from build123d import *

# Parameters (mm, degrees)
F1_W     = 9.5782261753
F1_H     = 9.891791337
F1_H_2   = 10.108208663
F1_W_2   = 10
F1_H_3   = 10
F2_DEPTH = 5
F3_W     = 10.1701691747
F3_H     = 1.1901259422
F3_W_2   = 2.3802500218
F3_W_3   = 1.1901250109
F3_H_2   = 0.8006438729
F3_H_3   = 10.4947462678
F3_W_4   = 5.1932781935
F3_H_4   = 1.9474774599
F3_W_5   = 1.1901259422
F3_H_5   = 8.5062488797
F3_W_6   = 9.7373928875
F3_W_7   = 1.514704898
F3_H_6   = 9.3068927526
F3_W_8   = 10.1330708712
F3_H_7   = 1.6025230289
F3_W_9   = 9.0882331133
F3_H_8   = 3.835350275
F3_W_10  = 1.0448377579
F3_H_9   = 8.595854044
F3_W_11  = 1.0108357528
F3_W_12  = 1.0278367554
F3_H_10  = 0.8937604725
F4_DEPTH = 25
F5_W     = 8.1058442593
F5_H     = 1.9299630076
F5_W_2   = 1.5439689159
F5_W_3   = 1.5439717099
F5_H_2   = 11.9657684118
F5_W_4   = 10.3005599231
F5_H_3   = 1.0513318703
F6_DEPTH = 25


# Not quite as in the source:
# - a feature names something its author has since deleted; it is built from what else it names


with BuildPart() as f2:
    # F1 (on Top) → F2 (new body)
    with BuildSketch(Plane.XY):
        with Locations((-4.7891130877, 4.9458956685)):
            Rectangle(F1_W, F1_H)
        Polygon((-10, 0), (-9.5782261753, 0), (-9.5782261753, 9.891791337), (-19.5782261753, 9.891791337), (-19.5782261753, 0), align=None)
        with Locations((-4.7891130877, 14.9458956685)):
            Rectangle(F1_W, F1_H_2)
        Polygon((0, 30), (0, 20), (0.4217738247, 20), (10, 20), (10, 30), align=None)
        Polygon((-9.5782261753, 20), (0, 20), (0, 30), (-10.0065707871, 30), align=None)
        with Locations((-24.5782261753, 4.9458956685)):
            Rectangle(F1_W_2, F1_H)
        with Locations((-24.5782261753, -5)):
            Rectangle(F1_W_2, F1_H_3)
        with BuildLine():
            Line((-10.0065707871, 30), (0, 30))
            Line((0, 30), (0, 44))
            ThreePointArc((0, 44), (-5.0363871882, 43.7108087787), (-10.0065707871, 42.8470365496))
            Line((-10.0065707871, 42.8470365496), (-10.0065707871, 30))
        make_face()
        with BuildLine():
            Line((-44, 0), (-29.5782261753, 0))
            Line((-29.5782261753, 0), (-29.5782261753, 9.891791337))
            add(Edge.make_bspline(
                [(-29.5782261753, 9.891791337), (-29.5956822452, 12.6865898133), (-29.4779762378, 16.6539770733), (-27.9306023487, 20)],
                knots=[0, 0, 0, 0, 0.3288616787, 0.3288616787, 0.3288616787, 0.3288616787], degree=3))
            Line((-27.9306023487, 20), (-39.1918358845, 20))
            ThreePointArc((-39.1918358845, 20), (-42.7810751321, 10.2849215136), (-44, 0))
        make_face()
        with BuildLine():
            add(Edge.make_bspline(
                [(-19.5782261753, 28.0459611928), (-16.4208018887, 29.540455447), (-13.1162348053, 30), (-10.0065707871, 30)],
                knots=[0.678814496, 0.678814496, 0.678814496, 0.678814496, 1, 1, 1, 1], degree=3))
            Line((-10.0065707871, 30), (-10.0065707871, 42.8470365496))
            ThreePointArc((-10.0065707871, 42.8470365496), (-14.8922224071, 41.4031606496), (-19.5782261753, 39.4042264209))
            Line((-19.5782261753, 39.4042264209), (-19.5782261753, 28.0459611928))
        make_face()
        with BuildLine():
            add(Edge.make_bspline(
                [(-24.5782261753, 24.6040217078), (-23.0917294817, 26.0318138691), (-21.358363516, 27.2033740757), (-19.5782261753, 28.0459611928)],
                knots=[0.497731988, 0.497731988, 0.497731988, 0.497731988, 0.678814496, 0.678814496, 0.678814496, 0.678814496], degree=3))
            Line((-19.5782261753, 28.0459611928), (-19.5782261753, 39.4042264209))
            ThreePointArc((-19.5782261753, 39.4042264209), (-23.9356591488, 36.9199704918), (-27.9820429197, 33.9559313529))
            Line((-27.9820429197, 33.9559313529), (-24.5782261753, 24.6040217078))
        make_face()
        with BuildLine():
            Line((-39.1918358845, 20), (-27.9306023487, 20))
            add(Edge.make_bspline(
                [(-27.9306023487, 20), (-27.136026622, 21.7181811177), (-25.9644735778, 23.2725198056), (-24.5782261753, 24.6040217078)],
                knots=[0.3288616787, 0.3288616787, 0.3288616787, 0.3288616787, 0.497731988, 0.497731988, 0.497731988, 0.497731988], degree=3))
            Line((-24.5782261753, 24.6040217078), (-33.9336129947, 28.00910404))
            ThreePointArc((-33.9336129947, 28.00910404), (-36.7813710365, 24.148100229), (-39.1918358845, 20))
        make_face()
        with BuildLine():
            Line((-33.9336129947, 28.00910404), (-24.5782261753, 24.6040217078))
            Line((-24.5782261753, 24.6040217078), (-27.9820429197, 33.9559313529))
            ThreePointArc((-27.9820429197, 33.9559313529), (-31.1002942205, 31.1250975806), (-33.9336129947, 28.00910404))
        make_face()
    extrude(amount=F2_DEPTH)

    # F3 (on offset) → F4 (cut)
    with BuildSketch(Plane.XY.offset(3)):
        Polygon((-33.0700390041, 9.3068927526), (-33.0700390041, 0), (-31.8799139932, 0), (-31.8799139932, 0.8006438729), (-30.6897889823, 0.8006438729), (-30.6897889823, 9.3068927526), align=None)
        with Locations((-38.1551235914, 9.9019557238)):
            Rectangle(F3_W, F3_H)
        with Locations((-31.8799139932, 9.9019557238)):
            Rectangle(F3_W_2, F3_H)
        with Locations((-31.2848514877, 0.4003219365)):
            Rectangle(F3_W_3, F3_H_2)
        Polygon((-30.6897889823, 0), (-31.8799139932, 0), (-31.8799139932, -0.8824482211), (-21.3851686567, -0.8824482211), (-21.3851686567, 0), (-22.5752945989, 0), (-22.5752945989, 0.8006438729), (-30.6897889823, 0.8006438729), align=None)
        with Locations((-31.8799139932, 15.7443918288)):
            Rectangle(F3_W_2, F3_H_3)
        with Locations((-35.6666781008, 21.9655036926)):
            Rectangle(F3_W_4, F3_H_4)
        Polygon((-33.0700390041, 22.9392424226), (-33.0700390041, 20.9917649627), (-30.6897889823, 20.9917649627), (-30.6897889823, 22.9392424226), (-31.3607603312, 22.9392424226), align=None)
        with Locations((-21.9802316278, 5.0537683128)):
            Rectangle(F3_W_5, F3_H_5)
        with Locations((-21.9802316278, 9.9019557238)):
            Rectangle(F3_W_5, F3_H)
        with Locations((-21.9802316278, 0.4003219365)):
            Rectangle(F3_W_5, F3_H_2)
        with Locations((-16.516472213, 9.9019557238)):
            Rectangle(F3_W_6, F3_H)
        Polygon((-29.9641676247, 26.1324569583), (-31.3607603312, 22.9392424226), (-30.6897889823, 22.9392424226), (-29.4176749885, 22.9392424226), (-28.3854100853, 25.160914287), (-27.413867414, 27.1647218615), (-25.7743895054, 28.682757169), (-24.2563541979, 29.8971850425), (-22.5752945989, 30.6865628809), (-22.5752945989, 31.9009907544), (-23.8920263946, 31.41522035), (-26.1387173086, 30.0793480128), (-26.8673747778, 29.40273819), (-26.8673747778, 27.7112144977), (-27.413867414, 27.7112144977), (-27.9603600502, 27.7112144977), (-28.6890175194, 27.7112144977), align=None)
        with Locations((-10.8904233202, 4.6534463763)):
            Rectangle(F3_W_7, F3_H_6)
        with Locations((-10.8904233202, 9.9019557238)):
            Rectangle(F3_W_7, F3_H)
        Polygon((-22.5752945989, 30.6865628809), (-22.5752945989, 22.9392424226), (-21.3851686567, 22.9392424226), (-21.3851686567, 33.2975834608), (-22.5752945989, 33.2975834608), (-22.5752945989, 31.9009907544), align=None)
        with Locations((-10.8904233202, 15.7443918288)):
            Rectangle(F3_W_7, F3_H_3)
        with Locations((-5.0665354356, 9.9019557238)):
            Rectangle(F3_W_8, F3_H)
        Polygon((-27.9603600502, 28.3878243205), (-28.6890175194, 27.7112144977), (-27.9603600502, 27.7112144977), align=None)
        Polygon((-33.9717790484, 27.7112144977), (-28.6890175194, 27.7112144977), (-27.9603600502, 28.3878243205), (-27.9603600502, 28.5613127053), (-33.9717790484, 28.5613127053), align=None)
        with Locations((-10.8904233202, 21.9655036926)):
            Rectangle(F3_W_7, F3_H_4)
        Polygon((-27.9603600502, 28.5613127053), (-27.9603600502, 28.3878243205), (-27.7735262161, 28.5613127053), align=None)
        with Locations((-21.9802316278, 34.0988449752)):
            Rectangle(F3_W_5, F3_H_7)
        with Locations((-16.516472213, 34.0988449752)):
            Rectangle(F3_W_6, F3_H_7)
        with Locations((-5.5889543146, 21.9655036926)):
            Rectangle(F3_W_9, F3_H_4)
        Polygon((-27.413867414, 28.5613127053), (-27.413867414, 27.7112144977), (-26.8673747778, 27.7112144977), (-26.8673747778, 29.40273819), (-27.7735262161, 28.5613127053), align=None)
        Polygon((-27.9603600502, 34.6941761672), (-27.9603600502, 28.5613127053), (-27.7735262161, 28.5613127053), (-26.8673747778, 29.40273819), (-26.8673747778, 34.6941761672), align=None)
        with Locations((-21.9802316278, 36.8177816272)):
            Rectangle(F3_W_5, F3_H_8)
        with Locations((-10.8904233202, 34.0988449752)):
            Rectangle(F3_W_7, F3_H_7)
        with Locations((-0.522418879, 21.9655036926)):
            Rectangle(F3_W_10, F3_H_4)
        with Locations((-10.8904233202, 39.1980335116)):
            Rectangle(F3_W_7, F3_H_9)
        Polygon((-10.1330708712, 34.9001064897), (-10.1330708712, 33.2975834608), (-1.0448377579, 33.2975834608), (-1.0448377579, 34.1913439333), (-0.0170010026, 34.1913439333), (-0.0170010026, 34.9001064897), align=None)
        Polygon((-1.0448377579, 33.2975834608), (-1.0448377579, 22.9392424226), (0, 22.9392424226), (1.0108357528, 22.9392424226), (1.0108357528, 34.1913439333), (-0.0170010026, 34.1913439333), (-0.0170010026, 33.2975834608), align=None)
        with Locations((0.5054178764, 21.9655036926)):
            Rectangle(F3_W_11, F3_H_4)
        with Locations((-0.5309193803, 33.7444636971)):
            Rectangle(F3_W_12, F3_H_10)
    extrude(amount=F4_DEPTH, mode=Mode.SUBTRACT)

    # F5 (on offset) → F6 (cut)
    with BuildSketch(Plane.XY.offset(3)):
        with Locations((-26.8084984273, 22.0622615889)):
            Rectangle(F5_W, F5_H)
        with Locations((-21.9835918397, 22.0622615889)):
            Rectangle(F5_W_2, F5_H)
        Polygon((-11.7547893897, 23.0272430927), (-21.2116073817, 23.0272430927), (-21.2116073817, 21.0972800851), (-10.2108176798, 21.0972800851), (-10.2108176798, 23.0272430927), align=None)
        Polygon((-21.2116073817, 21.0972800851), (-22.7555762976, 21.0972800851), (-22.7555762976, 10.4401707649), (-22.7555762976, 9.3888388947), (-21.2116073817, 9.3888388947), align=None)
        with Locations((-10.9828035347, 29.0101272985)):
            Rectangle(F5_W_3, F5_H_2)
        with Locations((-27.9058562592, 9.9145048298)):
            Rectangle(F5_W_4, F5_H_3)
    extrude(amount=F6_DEPTH, mode=Mode.SUBTRACT)


solid = f2.part
Work out the finished part from the listing and answer in its coordinate system (mm). A direction names the side the tool comes from. Give positions to 0.01 mm unless a question says otherwise; leave off trailing zeros. Loops run counter-clockwise (first coordinate to the right, second up) from the corner with the lowest first, then second, coordinate; pieces in that order, holes last. Notation, with made-up numbers: (-25.75, -38) - (17.25, -38) arc R22 cw to (17.25, -27) - close; hole circle Ø8 at (-10, -15.75). An arc over 180 degrees is marked (long way). Answer in a Markdown table with one row per item.
(1) Section D-D (y = 36) is taken. Give the vertices of the cut face in (x, z), and give its area (3 significant figures).
Results list:
| item | result |
|---|---|
| outline | (-25.3, 0) - (0, 0) - (0, 5) - (-10.13, 5) - (-10.13, 3) - (-11.65, 3) - (-11.65, 5) - (-21.39, 5) - (-21.39, 3) - (-22.58, 3) - (-22.58, 5) - (-25.3, 5) - close |
| area | 121 mm² |
(2) A tool of negligible diameter and unlimited length cuts with its end or side. For faces 4 (the face through (-9.795, 25.07, 2.465)), 5 (the face through (-37, 0, 2)), 6 (the face through (-27.906, 26.149, 3.986)), from which of +Z, -Z, +X, -X, +Y, -Y can it reach the whole face along a straight path? Write none if from no direction.
Results list:
| item | result |
|---|---|
| face 4 | +Z, -Z |
| face 5 | +Z, -Z, -X, -Y |
| face 6 | +Z |
(3) Consider L1, parallel to X at y = 5.5, z = 4.45; L2, parallel to X at y = 8.5, z = 4; L3, parallel to Y at x = -25.5, z = 3.2. Determine where each line is inside the solid, lowest interval first. Write a range as [from, to].
Results list:
| item | result |
|---|---|
| L1 | x = [-43.65, -33.07], [-30.69, -22.58], [-21.39, -11.65], [-10.13, 0] |
| L2 | x = [-43.17, -33.07], [-30.69, -22.58], [-21.39, -11.65], [-10.13, 0] |
| L3 | y = [-10, -0.88], [0.8, 9.39], [23.65, 28.9], [30.46, 35.86] |
(4) For a pull along Y with two mould halves and no side action, classify faces 1 (the face through (-28, 23.027, 4)), 2 (the face through (-25, -10, 2)), 3 (the face through (-22.575, 29, 4)) as pulls with the +Y half, pulls with the -Y half, needs draft (parallel to the pull), parting line crosses it, or undercut.
Results list:
| item | result |
|---|---|
| face 1 | undercut |
| face 2 | pulls with the -Y half |
| face 3 | needs draft |
(5) Section C-C (x = -8.5) is taken. Give the vertices of the cut face in (y, z), and give its area (3 significant figures).
Results list:
| item | result |
|---|---|
| outline | (0, 0) - (43.17, 0) - (43.17, 5) - (34.9, 5) - (34.9, 3) - (33.3, 3) - (33.3, 5) - (22.94, 5) - (22.94, 3) - (20.99, 3) - (20.99, 5) - (10.5, 5) - (10.5, 3) - (9.31, 3) - (9.31, 5) - (0, 5) - close |
| area | 206 mm² |
(6) Flat-ended cylindrical pins translate along their axes: pin 1 Ø1 at (x, z) = (-40.5, 4) entering from -Y; pin 2 Ø1 at (y, z) = (4, 4) entering from +X; pin 3 Ø2 at (y, z) = (30.5, 4) entering from -X. Find the tip coordinate at first contact, or state that the pin passes through.
Results list:
| item | result |
|---|---|
| pin 1 | stops at y = 0 |
| pin 2 | stops at x = 0 |
| pin 3 | stops at x = -32.65 |
(7) Section A-A (y = 8) is taken. Give the vertices of the cut face in (x, z).
Results list:
| item | result |
|---|---|
| outline | (-43.27, 0) - (0, 0) - (0, 5) - (-10.13, 5) - (-10.13, 3) - (-11.65, 3) - (-11.65, 5) - (-21.39, 5) - (-21.39, 3) - (-22.58, 3) - (-22.58, 5) - (-30.69, 5) - (-30.69, 3) - (-33.07, 3) - (-33.07, 5) - (-43.27, 5) - close |
(8) Section B-B (x = 2.5) is taken. Give the vertices of the cut face in (y, z), and give its area (3 significant figures).
Results list:
| item | result |
|---|---|
| outline | (20, 0) - (30, 0) - (30, 5) - (20, 5) - close |
| area | 50.0 mm² |
